```python
from build123d import *

# Parameters (mm, degrees)
SKETCH1_R           = 7.9375
SKETCH1_R_2         = 2.9845
SKETCH1_R_3         = 1.524
SKETCH1_R_4         = 7.250000001
BOSS_EXTRUDE1_DEPTH = 6.35
SKETCH1_3_R         = 7.9375
SKETCH1_3_R_2       = 7.250000001
CUT_EXTRUDE1_DEPTH  = 4.699


with BuildPart() as part:
    # Sketch1 → Boss-Extrude1 (new body)
    # profile 1 of 2: a face of its own
    with BuildSketch(Plane.XY):
        with BuildLine():
            Line((157.991701588, 172.208854223), (157.991701588, 205.858854223))
            ThreePointArc((157.991701588, 205.858854223), (157.061765618, 208.103918253), (154.816701588, 209.033854223))
            Line((154.816701588, 209.033854223), (131.166701588, 209.033854223))
            ThreePointArc((131.166701588, 209.033854223), (128.921637558, 208.103918253), (127.991701588, 205.858854223))
            Line((127.991701588, 205.858854223), (127.991701588, 172.208854223))
            ThreePointArc((127.991701588, 172.208854223), (128.921637558, 169.963790192), (131.166701588, 169.033854223))
            Line((131.166701588, 169.033854223), (154.816701588, 169.033854223))
            ThreePointArc((154.816701588, 169.033854223), (157.061765618, 169.963790192), (157.991701588, 172.208854223))
        make_face()
        with Locations((142.991701588, 199.033854223)):
            Circle(SKETCH1_R, mode=Mode.SUBTRACT)
        with Locations((150.991701587, 179.033854223)):
            Circle(SKETCH1_R_2, mode=Mode.SUBTRACT)
        with Locations((134.991701588, 179.033854223)):
            Circle(SKETCH1_R_2, mode=Mode.SUBTRACT)
        with Locations((153.786701588, 199.033854223)):
            Circle(SKETCH1_R_3, mode=Mode.SUBTRACT)
    # profile 2 of 2: a face of its own
    with BuildSketch(Plane.XY):
        with Locations((142.991701588, 199.033854223)):
            Circle(SKETCH1_R)
        with Locations((142.991701588, 199.033854223)):
            Circle(SKETCH1_R_4, mode=Mode.SUBTRACT)
    extrude(amount=BOSS_EXTRUDE1_DEPTH)

    # Sketch1_3 → Cut-Extrude1 (cut)
    with BuildSketch(Plane.XY):
        with Locations((142.991701588, 199.033854223)):
            Circle(SKETCH1_3_R)
        with Locations((142.991701588, 199.033854223)):
            Circle(SKETCH1_3_R_2, mode=Mode.SUBTRACT)
    extrude(amount=CUT_EXTRUDE1_DEPTH, mode=Mode.SUBTRACT)


solid = part.part
```
Read the model definition and answer for the solid it produces. Units are mm, in the model's axes. A direction names the side the tool comes from. Round coordinates to 2 decimals unless told otherwise and drop trailing zeros. Write each loop counter-clockwise with the first axis right and the second up, starting at its lowest first coordinate (ties: lowest second). Pieces come first, ordered by that corner, then holes. Notation, with made-up numbers: (67, 87.5) -> (107, 87.5) arc R14 cw to (107, 105.5) -> close; hole circle Ø6 at (65.5, -22.5). An arc over 180 degrees is marked (long way). Answer in a Markdown table with one row per item. Add a question column.
1) Find section B-B, the plane z = 3.25. State how many separate pieces and enclosed holes the cut face has, and give its area (3 significant figures).
2) Given P1, Ø8, axis at x = 139.5, y = 200, coming from the -Z side, flat-ended and moving along its own axis, determine where the tip first touches the part or whether it passes through.
3) Find section C-C, the plane x = 146.5. Determine the outline of the cut face in (y, z), and give its area (3 significant figures).
4) Find section A-A, the plane x = 140. Determine the outline of the cut face in (y, z).
5) Consider line 1 (Y direction, x = 151, z = 5.75); line 2 (X direction, y = 181, z = 4.75); line 3 (Y direction, x = 143, z = 1.25). Determine where each line is inside the solid, lowest interval first.
6) Which of the six approach directions +Z, -Z, +X, -X, +Y, -Y give full straight-line access (tool end or side, diameter ignored) to faces 1 (the face through (157.992, 189, 3)), 2 (the face through (137.141, 204.398, 2.317))?
7) Determine the mould class of faces 3 (the face through (143, 189, 6.35)), 4 (the face through (127.992, 189, 3)), 5 (the face through (145.3, 192, 4.699)) for opening direction X: pulls with the +X half, pulls with the -X half, needs draft (parallel to the pull), parting line crosses it, or undercut.
Findings below:
| question | item | result |
|---|---|---|
| 1 | separate pieces | 1 |
| 1 | enclosed holes | 4 |
| 1 | area | 930 mm² |
| 2 | P1 | z = 4.7 |
| 3 | outline | (169.03, 0) -> (191.91, 0) -> (191.91, 4.7) -> (192.69, 4.7) -> (192.69, 6.35) -> (169.03, 6.35) -> close; (205.38, 4.7) -> (206.15, 4.7) -> (206.15, 0) -> (209.03, 0) -> (209.03, 6.35) -> (205.38, 6.35) -> close |
| 3 | area | 166 mm² |
| 4 | outline | (169.03, 0) -> (191.68, 0) -> (191.68, 4.7) -> (192.43, 4.7) -> (192.43, 6.35) -> (169.03, 6.35) -> close; (205.64, 4.7) -> (206.39, 4.7) -> (206.39, 0) -> (209.03, 0) -> (209.03, 6.35) -> (205.64, 6.35) -> close |
| 5 | line 1 | 169.03 to 176.05, 182.02 to 209.03 |
| 5 | line 2 | 127.99 to 132.75, 137.24 to 148.75, 153.24 to 157.99 |
| 5 | line 3 | 169.03 to 191.1, 206.97 to 209.03 |
| 6 | face 1 | +Z, -Z, +X, +Y, -Y |
| 6 | face 2 | -Z |
| 7 | face 3 | needs draft |
| 7 | face 4 | pulls with the -X half |
| 7 | face 5 | undercut |
